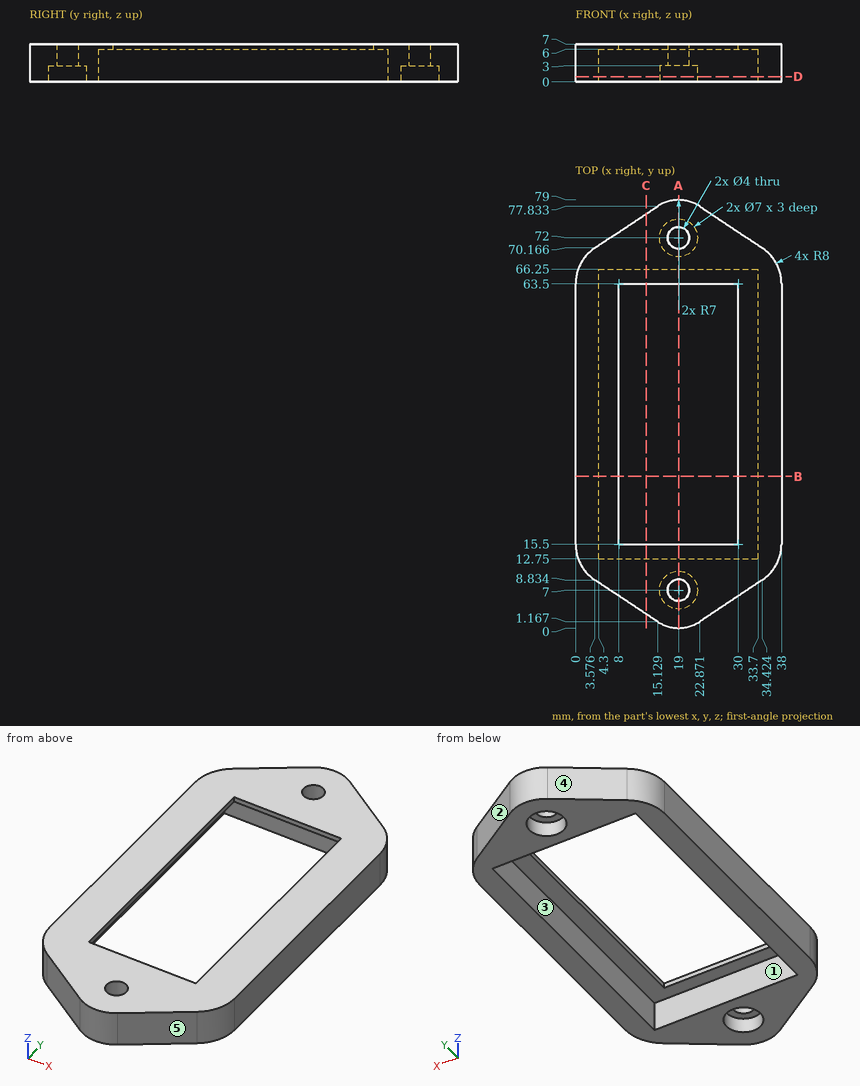
Geometry check sheet. Reference: drawing and pictorial views, mm from the part's lowest x, y, z. A direction names the side the tool comes from. Round coordinates to 2 decimals unless told otherwise and drop trailing zeros. Loops run counter-clockwise (first coordinate to the right, second up) from the corner with the lowest first, then second, coordinate; pieces in that order, holes last.
1. Sectioned sample at C-C on x = 13. Record the boundary of the cut face in (y, z).
2. Sectioned sample at A-A on x = 19. Record the boundary of the cut face in (y, z), and give its area (3 significant figures).
3. Gauge pin test, flat ends, axial feed: pin 1 Ø0.5 at (x, z) = (22, 6.5) entering from -Y; pin 2 Ø3 at (x, z) = (23.5, 4.5) entering from -Y (1 decimal); pin 3 Ø3 at (x, y) = (19, 7) entering from -Z. Record the tip position at first contact, or that the pin passes through.
4. Mould release check, pull along X, two halves, no side actions. Record for the marked faces 3, 4 and 5: released by +X, released by -X, zero draft, split by the parting line, or undercut.
5. Sectioned sample at D-D on z = 1. Give the number of separate pieces and of enclosed holes in the cut face.
6. Scan lines: probe 1 along Y at (x, z) = (19, 1.8); probe 2 along Y at (x, z) = (19, 4.3); probe 3 along X at (y, z) = (50, 3.5). Record each from-to range of solid material in increasing order.
7. Set-up check for the marked faces 1 and 2: record each of +Z, -Z, +X, -X, +Y, -Y from which the full face is reachable in a straight line by a thin tool's end or side.
8. Sectioned sample at B-B on y = 28. Record the boundary of the cut face in (x, z).
Recorded:
1. outline: (2.58, 0) - (12.75, 0) - (12.75, 6) - (15.5, 6) - (15.5, 7) - (2.58, 7) - close; (63.5, 6) - (66.25, 6) - (66.25, 0) - (76.42, 0) - (76.42, 7) - (63.5, 7) - close
2. outline: (0, 0) - (3.5, 0) - (3.5, 3) - (5, 3) - (5, 7) - (0, 7) - close; (9, 3) - (10.5, 3) - (10.5, 0) - (12.75, 0) - (12.75, 6) - (15.5, 6) - (15.5, 7) - (9, 7) - close; (63.5, 6) - (66.25, 6) - (66.25, 0) - (68.5, 0) - (68.5, 3) - (70, 3) - (70, 7) - (63.5, 7) - close; (74, 3) - (75.5, 3) - (75.5, 0) - (79, 0) - (79, 7) - (74, 7) - close
2. area: 110 mm2
3. pin 1: stops at y = 0.56
3. pin 2: stops at y = 0.7
3. pin 3: passes through
4. face 3: undercut
4. face 4: released by -X
4. face 5: released by +X
5. separate pieces: 1
5. enclosed holes: 3
6. probe 1: y = 0 to 3.5, 10.5 to 12.75, 66.25 to 68.5, 75.5 to 79
6. probe 2: y = 0 to 5, 9 to 12.75, 66.25 to 70, 74 to 79
6. probe 3: x = 0 to 4.3, 33.7 to 38
7. face 1: -Z
7. face 2: +Z, -Z, +X, +Y
8. outline: (0, 0) - (4.3, 0) - (4.3, 6) - (8, 6) - (8, 7) - (0, 7) - close; (30, 6) - (33.7, 6) - (33.7, 0) - (38, 0) - (38, 7) - (30, 7) - close
